```python
from build123d import *

# Parameters (mm, degrees)
F0_W     = 25
F0_H     = 25
F1_DEPTH = 60
F2_W     = 25
F2_H     = 25
F3_DEPTH = 60
F4_DEPTH = 25
F5_DEPTH = 50
F6_W     = 25
F6_H     = 25
F7_DEPTH = 110
F8_R     = 5


with BuildPart() as f1:
    # F0 (on Top) → F1 (new body)
    with BuildSketch(Plane.XY):
        with Locations((12.5, 12.5)):
            Rectangle(F0_W, F0_H)
    extrude(amount=F1_DEPTH)

    # F2 (on face) → F3 (join)
    with BuildSketch(Plane.YZ.offset(25)):
        with Locations((12.5, 47.5)):
            Rectangle(F2_W, F2_H)
    extrude(amount=F3_DEPTH)

    # F4 (add): a face of the model
    f4_faces = [f1.faces().sort_by_distance(p)[0] for p in [
        (12.5, 12.5, 0),
    ]]
    extrude(f4_faces, amount=F4_DEPTH)

    # F5 (add): a face of the model
    f5_faces = [f1.faces().sort_by_distance(p)[0] for p in [
        (85, 12.5, 47.5),
    ]]
    extrude(f5_faces, amount=F5_DEPTH)

    # F6 (on face) → F7 (join)
    with BuildSketch(Plane(origin=(0, 0, 35), x_dir=(1, 0, 0), z_dir=(0, 0, -1))):
        with Locations((122.5, -12.5)):
            Rectangle(F6_W, F6_H)
    extrude(amount=F7_DEPTH)

    # F8
    f8_edges = [f1.edges().sort_by_distance(p)[0] for p in [
        (67.5, 0, 60),
        (67.5, 25, 60),
        (25, 0, 5),
        (25, 25, 5),
        (0, 0, 17.5),
        (0, 25, 17.5),
        (67.5, 0, 35),
        (135, 0, -7.5),
        (135, 25, -7.5),
        (135, 12.5, 60),
        (0, 12.5, 60),
        (67.5, 25, 35),
        (110, 0, -20),
    ]]
    fillet(f8_edges, radius=F8_R)


solid = f1.part
```
Geometry: final body of the model. Coordinates: model frame, mm. A direction names the side the tool comes from. Coordinates: 2 decimals unless noted, no trailing zeros. Order: outer loops, then holes, each group sorted by start corner. A loop starts at its lowest first (then second) coordinate and runs counter-clockwise, first axis right, second up. Notation, with made-up numbers: (-22, -38.75) -> (-4, -38.75) arc R28 cw to (-4, 0.25) -> close; hole circle Ø8 at (1, -34). An arc over 180 degrees is marked (long way). Answer in a Markdown table with one row per item.
Item 1: Draft query along X for faces 1 (the cylindrical face through (2, 13, 59)), 2 (the cylindrical face through (134, 13, 58)), 3 (the flat face through (25, 12, 5)). Return one class per face: released by +X, released by -X, zero draft, split by the parting line, or undercut.
Return value:
| item | result |
|---|---|
| face 1 | released by -X |
| face 2 | released by +X |
| face 3 | undercut |
Item 2: Access query for faces 4 (the flat face through (67, 12, 35)), 5 (the cylindrical face through (66, 23, 36)), 6 (the cylindrical face through (68, 2, 36)). Directions: +Z, -Z, +X, -X, +Y, -Y. A direction counts if a zero-diameter tool reaches every point of the face in a straight line with its end or side. Return the directions, or none.
Return value:
| item | result |
|---|---|
| face 4 | -Z, +Y, -Y |
| face 5 | -Z, +Y |
| face 6 | -Z, -Y |
Item 3: Ray query, L1, parallel to X at y = 9.75, z = 13.5; L2, parallel to X at y = 18.25, z = -53; L3, parallel to Z at x = 66.5, y = 5. Return the intervals inside material, ascending.
Return value:
| item | result |
|---|---|
| L1 | x = 0 to 25, 110 to 135 |
| L2 | x = 110 to 135 |
| L3 | z = 35 to 60 |
Item 4: Section D-D on z = -27. Output: boundary loops of the cut face in (x, y), plus the area to 3 significant figures.
Return value:
| item | result |
|---|---|
| outline | (110, 5) arc R5 ccw to (115, 0) -> (130, 0) arc R5 ccw to (135, 5) -> (135, 20) arc R5 ccw to (130, 25) -> (110, 25) -> close |
| area | 609 mm² |
Item 5: Section C-C on x = 58. Output: boundary loops of the cut face in (y, z).
Return value:
| item | result |
|---|---|
| outline | (0, 40) arc R5 ccw to (5, 35) -> (20, 35) arc R5 ccw to (25, 40) -> (25, 55) arc R5 ccw to (20, 60) -> (5, 60) arc R5 ccw to (0, 55) -> close |
Item 6: Section A-A on z = -7. Output: boundary loops of the cut face in (x, y).
Return value:
| item | result |
|---|---|
| outline | (0, 5) arc R5 ccw to (5, 0) -> (20, 0) arc R5 ccw to (25, 5) -> (25, 20) arc R5 ccw to (20, 25) -> (5, 25) arc R5 ccw to (0, 20) -> close; (110, 5) arc R5 ccw to (115, 0) -> (130, 0) arc R5 ccw to (135, 5) -> (135, 20) arc R5 ccw to (130, 25) -> (110, 25) -> close |
Item 7: Contact query for flat-ended pins moving along their axis: P1, Ø2, axis at y = 20.5, z = 39, coming from the -X side; P2, Ø7.5, axis at x = 77.5, y = 11.5, coming from the -Z side; P3, Ø1, axis at x = 70, z = 36.5, coming from the +Y side; P4, Ø7.5, axis at x = 16.5, y = 13.5, coming from the -Z side. Output: stop coordinate, or through.
Return value:
| item | result |
|---|---|
| P1 | stops at x = 0 |
| P2 | stops at z = 35 |
| P3 | stops at y = 24 |
| P4 | stops at z = -25 |
Item 8: Section B-B on y = 11. Output: boundary loops of the cut face in (x, z), plus the area to 3 significant figures.
Return value:
| item | result |
|---|---|
| outline | (0, -25) -> (25, -25) -> (25, 35) -> (110, 35) -> (110, -75) -> (135, -75) -> (135, 55) arc R5 ccw to (130, 60) -> (5, 60) arc R5 ccw to (0, 55) -> close |
| area | 7,610 mm² |
